Read the model definition and answer for the solid it produces. Units are mm, in the model's axes. A direction names the side the tool comes from. Round coordinates to 2 decimals unless told otherwise and drop trailing zeros. Order: outer loops, then holes, each group sorted by start corner. A loop starts at its lowest first (then second) coordinate and runs counter-clockwise, first axis right, second up. Notation, with made-up numbers: (66.5, 59.25) -> (81.5, 59.25) arc R26 ccw to (81.5, 75.25) -> close; hole circle Ø3 at (15, -39). An arc over 180 degrees is marked (long way). One line per item, written item: value. Start each with the question number.
1. For faces 1 (the face through (12.36, 3.89, 12.26)), 2 (the face through (0, 4, 10)), 3 (the face through (25.654, 4, 10)), determine the directions among +Z, -Z, +X, -X, +Y, -Y from which every point of the face is accessible in a straight line to the end or side of a thin tool.
2. Section D-D (y = 33.5) is taken. Give the vertices of the cut face in (x, z), then the cut area to 3 significant figures.
3. The mould has two halves that part along X. Classify faces 4 (the face through (13, 7, 20.32)), 5 (the face through (19.91, 16.97, 10.02)), 6 (the face through (13.132, 39.925, 10.018)): released by +X, released by -X, zero draft, split by the parting line, or undercut.
4. Section B-B (x = 7.5) is taken. Give the vertices of the cut face in (y, z), then the cut area to 3 significant figures.
5. Section A-A (z = 16.75) is taken. Give the vertices of the cut face in (x, y), then the cut area to 3 significant figures.
6. Consider line 1 (Y direction, x = 20.25, z = 10.5); line 2 (X direction, y = 2.5, z = 10.16); line 3 (Y direction, x = 22.5, z = 1.5). Determine where each line is inside the solid, lowest interval first.
7. Section C-C (x = 4.5) is taken. Give the vertices of the cut face in (y, z), then the cut area to 3 significant figures.
8. Flat-ended cylindrical pins translate along their axes: pin 1 Ø2.5 at (y, z) = (4.5, 14.5) entering from -X; pin 2 Ø4 at (y, z) = (4.5, 13.5) entering from +X. Find the tip coordinate at first contact, or state that the pin passes through.
from build123d import *

# Parameters (mm, degrees)
BOSS_EXTRUDE1_DEPTH       = 20.32
F_8_CLEARANCE_HOLE1_D     = 4.3053
F_8_CLEARANCE_HOLE1_DEPTH = 7.679166788


with BuildPart() as part:
    # Sketch1 → Boss-Extrude1 (new body)
    with BuildSketch(Plane.XY):
        with BuildLine():
            Line((0, 0), (25.654, 0))
            Line((25.654, 0), (25.654, 8.89))
            Line((25.654, 8.89), (26.081819356, 26.345128821))
            ThreePointArc((26.081819356, 26.345128821), (12.835928023, 39.928796994), (-0.42824485, 26.362979796))
            Line((-0.42824485, 26.362979796), (0, 7.874))
            Line((0, 7.874), (0, 0))
        make_face()
        with BuildLine():
            Line((2.545194005, 7.679166788), (23.083560079, 7.679166788))
            Line((23.083560079, 7.679166788), (23.351364853, 18.605663581))
            ThreePointArc((23.351364853, 18.605663581), (22.092748432, 17.18624107), (20.64444443, 15.960969231))
            Line((20.64444443, 15.960969231), (19.146849712, 18.012507692))
            ThreePointArc((19.146849712, 18.012507692), (12.827, 37.3888), (6.507150288, 18.012507692))
            Line((6.507150288, 18.012507692), (5.00955557, 15.960969231))
            ThreePointArc((5.00955557, 15.960969231), (3.55486763, 17.192482458), (2.291784196, 18.619844386))
            Line((2.291784196, 18.619844386), (2.545194005, 7.679166788))
        make_face(mode=Mode.SUBTRACT)
    extrude(amount=BOSS_EXTRUDE1_DEPTH)

    # #8 Clearance Hole1
    with Locations(Plane(origin=(0, 0, 0), x_dir=(-1, 0, 0), z_dir=(0, -1, 0))):
        with Locations((-12.827, -10.16)):
            Hole(F_8_CLEARANCE_HOLE1_D / 2, depth=F_8_CLEARANCE_HOLE1_DEPTH)


solid = part.part
Answer:
1. face 1: -Y
1. face 2: +Z, -Z, -X, -Y
1. face 3: +Z, -Z, +X, -Y
2. outline: (1.46, 0) -> (4.57, 0) -> (4.57, 20.32) -> (1.46, 20.32) -> close; (21.09, 0) -> (24.19, 0) -> (24.19, 20.32) -> (21.09, 20.32) -> close
2. area: 126 mm^2
3. face 4: zero draft
3. face 5: undercut
3. face 6: split by the parting line
4. outline: (0, 0) -> (7.68, 0) -> (7.68, 20.32) -> (0, 20.32) -> close; (35.97, 0) -> (38.81, 0) -> (38.81, 20.32) -> (35.97, 20.32) -> close
4. area: 214 mm^2
5. outline: (-0.43, 26.36) -> (0, 7.87) -> (0, 0) -> (25.65, 0) -> (25.65, 8.89) -> (26.08, 26.35) arc R13.26 ccw (long way) to start; hole (2.29, 18.62) -> (2.55, 7.68) -> (23.08, 7.68) -> (23.35, 18.61) arc R13.26 cw to (20.64, 15.96) -> (19.15, 18.01) arc R10.72 ccw (long way) to (6.51, 18.01) -> (5.01, 15.96) arc R13.26 cw to start
5. area: 418 mm^2
6. line 1: 0 to 7.68, 16.5 to 18.94, 34.4 to 37.66
6. line 2: 0 to 10.67, 14.98 to 25.65
6. line 3: 0 to 7.68, 17.6 to 22.05, 31.29 to 35.74
7. outline: (0, 0) -> (7.68, 0) -> (7.68, 20.32) -> (0, 20.32) -> close; (16.35, 0) -> (19.92, 0) -> (19.92, 20.32) -> (16.35, 20.32) -> close; (33.42, 0) -> (36.99, 0) -> (36.99, 20.32) -> (33.42, 20.32) -> close
7. area: 301 mm^2
8. pin 1: x = 0
8. pin 2: x = 25.65
